```python
from build123d import *

# Parameters (mm, degrees)
SKETCH_1_W           = 52
SKETCH_1_H           = 25
SKETCH_1_R           = 1.5
EXTRUDE_1_DEPTH      = 5
SKETCH_2_R           = 4
SKETCH_2_R_2         = 2.5
EXTRUDE_2_DEPTH      = 125
FILLET_1_R           = 10
SKETCH_2_3_R         = 6
SKETCH_2_3_R_2       = 4
EXTRUDE_4_DEPTH      = 125
FILLET_3_R           = 5
CUT_EXTRUDE_START    = -50
SKETCH_2_4_R         = 6
CUT_EXTRUDE_1_DEPTH  = 50
FILLET_4_R           = 5
EXTRUDE_5_DEPTH      = 23
EXTRUDE_5_DEPTH_BACK = 10
SKETCH_3_W           = 36.659715442
SKETCH_3_H           = 13
SKETCH_4_W           = 12.2
SKETCH_4_H           = 10.2
CUT_EXTRUDE_2_DEPTH  = 16
FILLET_5_R           = 10
EXTRUDE_6_DEPTH      = 8
FILLET_7_R           = 10
FILLET_8_R           = 10
SKETCH_9_R           = 9
SKETCH_9_R_2         = 2.5
CUT_EXTRUDE_4_DEPTH  = 35
SKETCH_10_W          = 48.137224848
SKETCH_10_H          = 8
EXTRUDE_9_DEPTH      = 2
FILLET_9_R           = 5
CUT_EXTRUDE_5_REACH  = 178.626
SKETCH_8_R           = 2
CUT_EXTRUDE_6_REACH  = 149.735
SKETCH_11_W          = 37.875915136
SKETCH_11_H          = 13.1
EXTRUDE_START        = 1
EXTRUDE_10_DEPTH     = 1
CUT_EXTRUDE_7_REACH  = 178.857
SKETCH_13_R          = 1.5
CUT_EXTRUDE_8_DEPTH  = 4
FILLET_11_R          = 4
SKETCH_16_R          = 1.25
CUT_EXTRUDE_10_DEPTH = 4


# Some blends are built 0.0001 mm under size
with BuildPart() as part:
    # 草图1 → 凸台-拉伸1 (new body)
    with BuildSketch(Plane(origin=(0, 0, 0), x_dir=(1, 0, 0), z_dir=(0, 1, 0))):
        Rectangle(SKETCH_1_W, SKETCH_1_H)
        with Locations(Location((-18.5, 0, 0), (0, 0, 270))):
            Circle(SKETCH_1_R, mode=Mode.SUBTRACT)
        with Locations(Location((18.5, 0, 0), (0, 0, 270))):
            Circle(SKETCH_1_R, mode=Mode.SUBTRACT)
    extrude(amount=EXTRUDE_1_DEPTH)

    # 草图2 → 凸台-拉伸2 (add)
    with BuildSketch(Plane.XZ):
        with Locations(Location((0, 0, 0), (0, 0, 90))):
            Circle(SKETCH_2_R)
        with Locations(Location((0, 0, 0), (0, 0, 270))):
            Circle(SKETCH_2_R_2, mode=Mode.SUBTRACT)
    extrude(amount=EXTRUDE_2_DEPTH)

    # 圆角1
    fillet_1_edges = [part.edges().sort_by_distance(p)[0] for p in [
        (26, 2.5, 12.5),
        (-26, 2.5, 12.5),
        (-26, 2.5, -12.5),
        (26, 2.5, -12.5),
    ]]
    fillet(fillet_1_edges, radius=FILLET_1_R)

    # 草图2<3> → 凸台-拉伸4 (add)
    with BuildSketch(Plane.XZ):
        with Locations(Location((0, 0, 0), (0, 0, 90))):
            Circle(SKETCH_2_3_R)
        Circle(SKETCH_2_3_R_2, mode=Mode.SUBTRACT)
    extrude(amount=EXTRUDE_4_DEPTH)

    # 圆角3
    fillet_3_edges = [part.edges().sort_by_distance(p)[0] for p in [
        (0, 0, -6),
    ]]
    fillet(fillet_3_edges, radius=FILLET_3_R)

    # 草图2<4> → 切除-拉伸1 (cut)
    with BuildSketch(Plane.XZ.offset(CUT_EXTRUDE_START)):
        with Locations(Location((0, 0, 0), (0, 0, 90))):
            Circle(SKETCH_2_4_R)
    extrude(amount=CUT_EXTRUDE_1_DEPTH, mode=Mode.SUBTRACT)

    # 圆角4
    # the kernel refuses this fillet: 5 mm, written as the material it adds along each edge
    with BuildSketch(Plane(origin=(0, 0, 0), x_dir=(0, 0, 1), z_dir=(1, 0, 0))) as fillet_4_piece_1:
        with BuildLine():
            CenterArc((1, -4.769696007), FILLET_4_R, 0, 72.542396876)
            Line((2.5, 0), (2.53, 0.09539392))
            ThreePointArc((2.53, 0.09539392), (4.25, 0.1), (6, 0.1))
            Line((6, 0.1), (6.1, 0))
            Line((6.1, 0), (6.1, -4.769696007))
            Line((6.1, -4.769696007), (6, -4.769696007))
        make_face()
    revolve(axis=Axis((0, 0, 0), (0, -1, 0)))

    # 草图3 → 凸台-拉伸5 (add, two sides: drawn at the far end of the back side and taken through both)
    with BuildSketch(Plane.XY.offset(-EXTRUDE_5_DEPTH_BACK)):
        with Locations((0, -131.5)):
            Rectangle(SKETCH_3_W, SKETCH_3_H)
    extrude(amount=EXTRUDE_5_DEPTH + EXTRUDE_5_DEPTH_BACK)

    # 草图4 → 切除-拉伸2 (cut)
    with BuildSketch(Plane(origin=(0, -125, 0), x_dir=(1, 0, 0), z_dir=(0, 1, 0))):
        with Locations((0, -15)):
            Rectangle(SKETCH_4_W, SKETCH_4_H)
    extrude(amount=-CUT_EXTRUDE_2_DEPTH, mode=Mode.SUBTRACT)

    # 圆角5
    fillet_5_edges = [part.edges().sort_by_distance(p)[0] for p in [
        (18.329857721, -131.5, -10),
        (-18.329857721, -131.5, -10),
        (18.329857721, -131.5, 23),
        (-18.329857721, -131.5, 23),
    ]]
    fillet(fillet_5_edges, radius=FILLET_5_R)

    # 草图5 → 凸台-拉伸6 (add)
    with BuildSketch(Plane.XY):
        Polygon((-18.329857721, -138), (-28.399053295, -150), (-28.399053295, -165), (-23.780251142, -173), (0.468760608, -173), (24.356973706, -173), (29.111967808, -164.22974568), (28.710245061, -149.235126017), (18.329857721, -138), align=None)
    extrude(amount=EXTRUDE_6_DEPTH)

    # 圆角7
    # the kernel refuses this fillet: 10 mm, written as the material it adds along each edge
    with BuildSketch(Plane(origin=(18.329857721, -138, 8), x_dir=(0, 1, 0), z_dir=(0, 0, -1))) as fillet_7_piece_1:
        with BuildLine():
            CenterArc((FILLET_7_R * 0.39124696726, FILLET_7_R), FILLET_7_R, 227.264457783, 42.735542217)
            Line((-FILLET_7_R * 0.287368460715, FILLET_7_R * 0.265506228132), (0, 0))
            Line((0, 0), (FILLET_7_R * 0.39124696726, 0))
        make_face()
    extrude(amount=8)
    with BuildSketch(Plane(origin=(-18.329857721, -138, 0), x_dir=(0, 1, 0), z_dir=(0, 0, 1))) as fillet_7_piece_2:
        with BuildLine():
            CenterArc((FILLET_7_R * 0.363970234266, FILLET_7_R), FILLET_7_R, 230, 40)
            Line((-FILLET_7_R * 0.27881737542, FILLET_7_R * 0.233955556881), (0, 0))
            Line((0, 0), (FILLET_7_R * 0.363970234266, 0))
        make_face()
    extrude(amount=8)

    # 圆角8
    fillet_8_edges = [part.edges().sort_by_distance(p)[0] for p in [
        (0, -138, 0),
    ]]
    fillet(fillet_8_edges, radius=FILLET_8_R - 0.0001)  # a hair under: the kernel refuses the full size

    # 草图9 → 切除-拉伸4 (cut)
    with BuildSketch(Plane.XZ.offset(173)):
        with Locations((-0.1, 14.9)):
            Circle(SKETCH_9_R)
        with Locations((-0.1, 14.9)):
            Circle(SKETCH_9_R_2, mode=Mode.SUBTRACT)
    extrude(amount=-CUT_EXTRUDE_4_DEPTH, mode=Mode.SUBTRACT)

    # 草图10 → 凸台-拉伸9 (add)
    with BuildSketch(Plane.XZ.offset(173)):
        with Locations((0.288361282, 4)):
            Rectangle(SKETCH_10_W, SKETCH_10_H)
    extrude(amount=-EXTRUDE_9_DEPTH)

    # 圆角9
    fillet_9_edges = [part.edges().sort_by_distance(p)[0] for p in [
        (0, -125, -6),
    ]]
    fillet(fillet_9_edges, radius=FILLET_9_R)

    # 草图8 → 切除-拉伸5 (cut, up to next)
    with BuildSketch(Plane.XY.offset(8), mode=Mode.PRIVATE) as cut_extrude_5_sk1:
        with Locations((23.25, -156.732435849)):
            Circle(SKETCH_8_R)
    cut_extrude_5_tool1 = extrude(cut_extrude_5_sk1.sketch, amount=-CUT_EXTRUDE_5_REACH, mode=Mode.PRIVATE) & part.part
    # 草图8 → 切除-拉伸5 (cut, up to next)
    with BuildSketch(Plane.XY.offset(8), mode=Mode.PRIVATE) as cut_extrude_5_sk2:
        with Locations((-23.25, -156.732435849)):
            Circle(SKETCH_8_R)
    cut_extrude_5_tool2 = extrude(cut_extrude_5_sk2.sketch, amount=-CUT_EXTRUDE_5_REACH, mode=Mode.PRIVATE) & part.part
    add(cut_extrude_5_tool1.solids().sort_by_distance((23.25, -156.732436, 8))[0], mode=Mode.SUBTRACT)
    add(cut_extrude_5_tool2.solids().sort_by_distance((-23.25, -156.732436, 8))[0], mode=Mode.SUBTRACT)

    # 草图11 → 切除-拉伸6 (cut, up to next)
    with BuildSketch(Plane.XZ.offset(138), mode=Mode.PRIVATE) as cut_extrude_6_sk1:
        with Locations((-0.053616604, 16.45)):
            Rectangle(SKETCH_11_W, SKETCH_11_H)
    cut_extrude_6_tool1 = extrude(cut_extrude_6_sk1.sketch, amount=-CUT_EXTRUDE_6_REACH, mode=Mode.PRIVATE) & part.part
    add(cut_extrude_6_tool1.solids().sort_by_distance((-0.053617, -138, 16.45))[0], mode=Mode.SUBTRACT)

    # 草图12 → 凸台-拉伸10 (add)
    with BuildSketch(Plane.XZ.offset(138).offset(EXTRUDE_START)):
        with BuildLine():
            Line((18.329857721, 9.9), (-18.329857721, 9.9))
            Line((-18.329857721, 9.9), (-18.329857721, 8))
            Line((-18.329857721, 8), (-5.878408085, 8))
            ThreePointArc((-5.878408085, 8), (-0.1, 5.9), (5.678408085, 8))
            Line((5.678408085, 8), (18.329857721, 8))
            Line((18.329857721, 8), (18.329857721, 9.9))
        make_face()
    extrude(amount=-EXTRUDE_10_DEPTH)

    # 草图13 → 切除-拉伸7 (cut, up to next)
    with BuildSketch(Plane.XY.offset(9.9), mode=Mode.PRIVATE) as cut_extrude_7_sk1:
        with Locations((-8.8, -129)):
            Circle(SKETCH_13_R)
    cut_extrude_7_tool1 = extrude(cut_extrude_7_sk1.sketch, amount=-CUT_EXTRUDE_7_REACH, mode=Mode.PRIVATE) & part.part
    # 草图13 → 切除-拉伸7 (cut, up to next)
    with BuildSketch(Plane.XY.offset(9.9), mode=Mode.PRIVATE) as cut_extrude_7_sk2:
        with Locations((8.8, -129)):
            Circle(SKETCH_13_R)
    cut_extrude_7_tool2 = extrude(cut_extrude_7_sk2.sketch, amount=-CUT_EXTRUDE_7_REACH, mode=Mode.PRIVATE) & part.part
    add(cut_extrude_7_tool1.solids().sort_by_distance((-8.8, -129, 9.9))[0], mode=Mode.SUBTRACT)
    add(cut_extrude_7_tool2.solids().sort_by_distance((8.8, -129, 9.9))[0], mode=Mode.SUBTRACT)

    # 草图14 → 切除-拉伸8 (cut)
    with BuildSketch(Plane(origin=(0, 0, -10), x_dir=(-1, 0, 0), z_dir=(0, 0, -1))):
        Polygon((-6.05, -130.58771324), (-6.05, -127.41228676), (-8.8, -125.824573519), (-11.55, -127.41228676), (-11.55, -130.58771324), (-8.8, -132.175426481), align=None)
        Polygon((6.05, -130.58771324), (6.05, -127.41228676), (8.8, -125.824573519), (11.55, -127.41228676), (11.55, -130.58771324), (8.8, -132.175426481), align=None)
    extrude(amount=-CUT_EXTRUDE_8_DEPTH, mode=Mode.SUBTRACT)

    # 圆角11
    fillet_11_edges = [part.edges().sort_by_distance(p)[0] for p in [
        (18.329857721, -139, 8.95),
        (-18.329857721, -139, 8.95),
    ]]
    fillet(fillet_11_edges, radius=FILLET_11_R)

    # 草图16 → 切除-拉伸10 (cut)
    with BuildSketch(Plane(origin=(0, 0, 0), x_dir=(-1, 0, 0), z_dir=(0, 0, -1))):
        with Locations((-5.288361282, -167)):
            Circle(SKETCH_16_R)
        with Locations(Location((4.711638718, -167, 0), (0, 0, 180))):
            Circle(SKETCH_16_R)
    extrude(amount=-CUT_EXTRUDE_10_DEPTH, mode=Mode.SUBTRACT)


solid = part.part
```
Design review of the part built by this model. Coordinates are the model's own, in mm. A direction names the side the tool comes from. Give positions to 0.01 mm unless a question says otherwise; leave off trailing zeros. Write each loop counter-clockwise with the first axis right and the second up, starting at its lowest first coordinate (ties: lowest second). Pieces come first, ordered by that corner, then holes.
(1) Add section A-A (y = -88). Give the boundary of the cut face in (x, z).
Checked values:
outline: circle Ø12 at (0, 0); hole circle Ø5 at (0, 0)
(2) Tool access review of faces 1 (the face through (-17.235, 2.465, 0.806)), 2 (the face through (-6.05, -129, -8)), 3 (the face through (-24.48, -145.33, 3.94)): name each direction out of +Z, -Z, +X, -X, +Y, -Y from which nothing blocks a thin tool from reaching the whole face with its end or side.
Checked values:
face 1: +Y
face 2: -Z
face 3: +Z, -Z, -X
(3) Clearance check with flat-ended pins moving along their axes: pin 1 Ø3 at (x, y) = (5, -167.5) entering from -Z; pin 2 Ø4 at (x, z) = (-0.5, -1) entering from +Y; pin 3 Ø15.5 at (x, y) = (6.5, -131) entering from +Z; pin 4 Ø3 at (x, y) = (-23.25, -156.73) entering from +Z. State where each tip first meets the part, or that it passes through.
Checked values:
pin 1: stops at z = 0
pin 2: stops at y = 0.24
pin 3: stops at z = 9.9
pin 4: passes through
(4) Mouldability with a two-part tool opening along Y and no side actions: class faces 4 (the face through (6, -158, 8)), 5 (the face through (0, -173, 4)), 6 (the face through (2.3, -61.76, 5.54)) as +Y half, -Y half, draft (parallel to the pull), parting line (faces both ways), or undercut.
Checked values:
face 4: draft
face 5: -Y half
face 6: undercut
(5) Wall thickness on line 1 along X through (y, z) = (4.9, 0); line 2 along X through (y, z) = (-129, 6.25); line 3 along Y through (x, z) = (-6, -9.5): over which ranges is each line inside the solid? List them lowest first.
Checked values:
line 1: x = -26 to -20, -17 to -6, 6 to 17, 20 to 26
line 2: x = -18.33 to -10.3, -7.3 to 7.3, 10.3 to 18.33
line 3: y = -138.01 to -125, 0 to 5
